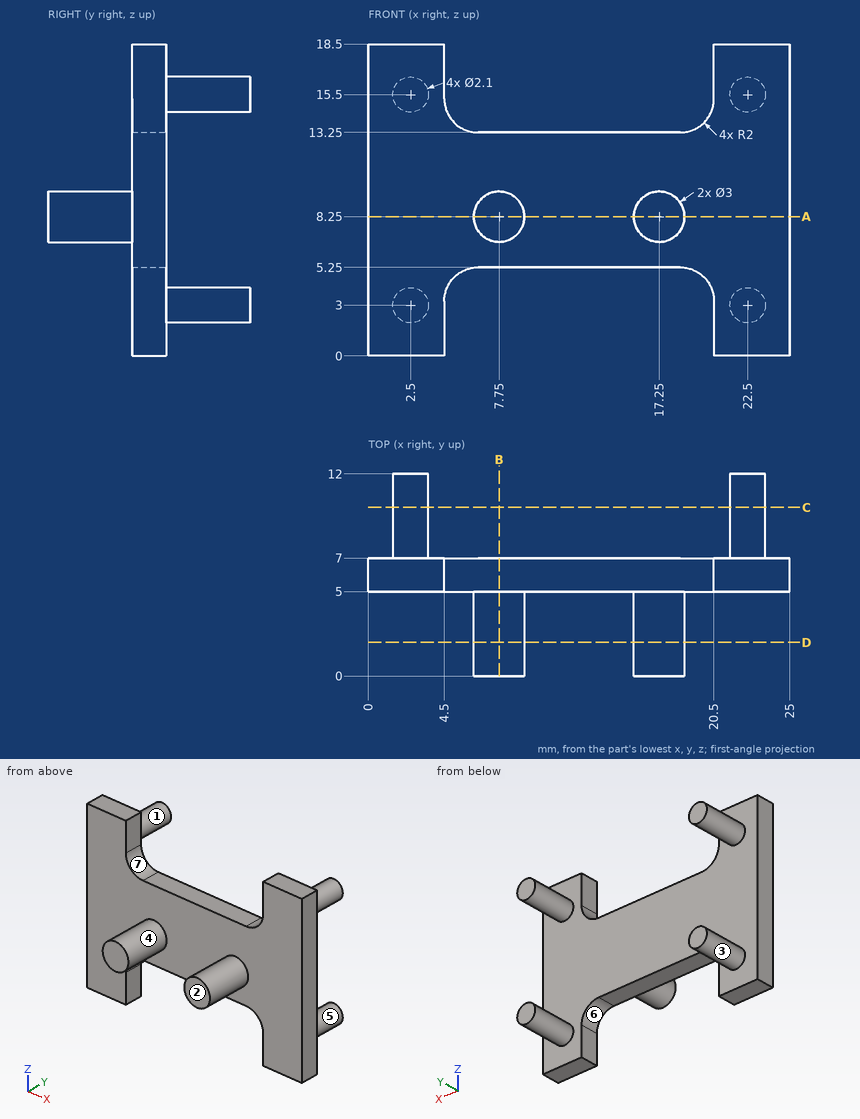
Source: three-view drawing plus pictorial views. Frame: mm from the lowest corner of the part. A direction names the side the tool comes from. Coordinates: 2 decimals unless noted, no trailing zeros. Order: outer loops, then holes, each group sorted by start corner. A loop starts at its lowest first (then second) coordinate and runs counter-clockwise, first axis right, second up. Notation, with made-up numbers: (76, 4.25) -> (122, 4.25) arc R12 cw to (122, 8.25) -> close; hole circle Ø5 at (65.5, -3). An arc over 180 degrees is marked (long way). Write item = value, one per line.
(1) Cut plane A-A on z = 8.25. Return loops of the section in (x, y), plus the area to 3 significant figures.
Solved:
outline = (0, 5) -> (6.25, 5) -> (6.25, 0) -> (9.25, 0) -> (9.25, 5) -> (15.75, 5) -> (15.75, 0) -> (18.75, 0) -> (18.75, 5) -> (25, 5) -> (25, 7) -> (0, 7) -> close
area = 80.0 mm²
(2) Access query for the marked faces 5, 6 and 7. Directions: +Z, -Z, +X, -X, +Y, -Y. A direction counts if a zero-diameter tool reaches every point of the face in a straight line with its end or side. Return the directions, or none.
Solved:
face_5 = +Y
face_6 = -Z, +Y, -Y
face_7 = +Z, +Y, -Y
(3) Cut plane B-B on x = 7.75. Return loops of the section in (y, z), plus the area to 3 significant figures.
Solved:
outline = (0, 6.75) -> (5, 6.75) -> (5, 5.25) -> (7, 5.25) -> (7, 13.25) -> (5, 13.25) -> (5, 9.75) -> (0, 9.75) -> close
area = 31.0 mm²
(4) Line query: line 1 (Y direction, x = 13.25, z = 5.5); line 2 (Y direction, x = 8, z = 9); line 3 (Z direction, x = 22, y = 7.5). Output: solid intervals per line, ascending.
Solved:
line_1 = 5 to 7
line_2 = 0 to 7
line_3 = 2.08 to 3.92, 14.58 to 16.42
(5) Cut plane C-C on y = 10. Return loops of the section in (x, z).
Solved:
outline = circle Ø2.1 at (2.5, 3); circle Ø2.1 at (2.5, 15.5); circle Ø2.1 at (22.5, 3); circle Ø2.1 at (22.5, 15.5)
(6) Pin query (flat end, axial travel): pin 1 Ø1 at (x, y) = (17, 6.5) entering from +Z; pin 2 Ø3 at (y, z) = (10.5, 12) entering from +X; pin 3 Ø9 at (x, z) = (6.5, 5) entering from +Y; pin 4 Ø1 at (x, y) = (15, 6) entering from -Z. Return the tip coordinate at first contact, or that it passes through.
Solved:
pin_1 = 13.25
pin_2 = through
pin_3 = 12
pin_4 = 5.25
(7) Cut plane D-D on y = 2. Return loops of the section in (x, z).
Solved:
outline = circle Ø3 at (7.75, 8.25); circle Ø3 at (17.25, 8.25)
(8) Pull-direction query (Z, two-part tool) for the marked faces 1, 2, 3 and 4; classes: pulls with the +Z half, pulls with the -Z half, needs draft (parallel to the pull), parting line crosses it, or undercut.
Solved:
face_1 = undercut
face_2 = needs draft
face_3 = undercut
face_4 = parting line crosses it
